Geometry: see drawing. Coordinates: mm, zero at the bounding-box minimum. Coordinates: 2 decimals unless noted, no trailing zeros. Loops run counter-clockwise (first coordinate to the right, second up) from the corner with the lowest first, then second, coordinate; pieces in that order, holes last. Notation, with made-up numbers: (3.25, 4.25) - (54.25, 4.25) arc R24 cw to (54.25, 33.25) - close; hole circle Ø1 at (16, 14). An arc over 180 degrees is marked (long way). Use one line per item in the form item = value.
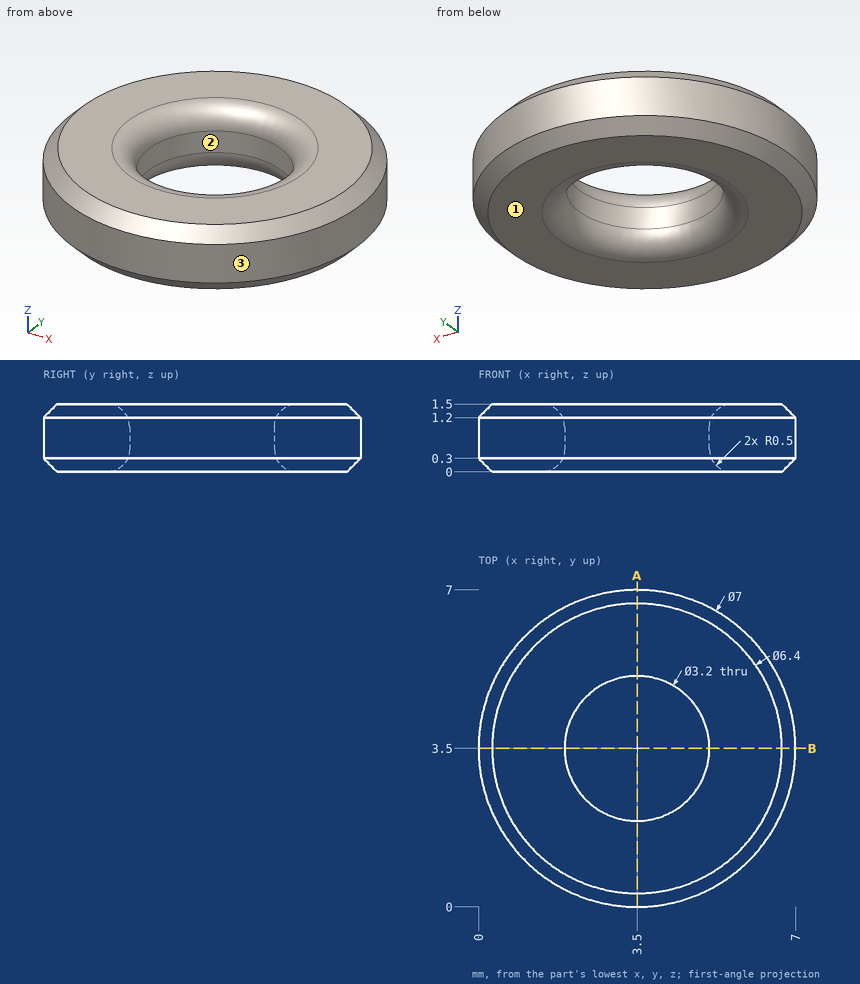
Q1. Cut plane A-A, the plane x = 3.5. Return loops of the section in (y, z), then the cut area to 3 significant figures.
Check values:
outline = (0, 0.3) - (0.3, 0) - (1.4, 0) arc R0.5 ccw to (1.9, 0.5) - (1.9, 1) arc R0.5 ccw to (1.4, 1.5) - (0.3, 1.5) - (0, 1.2) - close; (5.1, 0.5) arc R0.5 ccw to (5.6, 0) - (6.7, 0) - (7, 0.3) - (7, 1.2) - (6.7, 1.5) - (5.6, 1.5) arc R0.5 ccw to (5.1, 1) - close
area = 5.31 mm²
Q2. Pull-direction query (Y, two-part tool) for the marked faces 1, 2 and 3; classes: pulls with the +Y half, pulls with the -Y half, needs draft (parallel to the pull), parting line crosses it, or undercut.
Check values:
face_1 = needs draft
face_2 = undercut
face_3 = parting line crosses it
Q3. First-contact query: P1, Ø2.5, axis at x = 3.5, y = 3.5, coming from the +Z side. Flat tip, straight axial feed; report the tip coordinate or a pass-through.
Check values:
P1 = through
Q4. Ray query, line 1 along Y through (x, z) = (3.5, 0.8); line 2 along Y through (x, z) = (4.25, 0.4); line 3 along Z through (x, y) = (5.5, 3). Return the intervals inside material, ascending. Write a range as [from, to].
Check values:
line_1 = [0, 1.9], [5.1, 7]
line_2 = [0.08, 2.08], [4.92, 6.92]
line_3 = [0, 1.5]
